Part model, mm, in its own coordinate system. Face numbers are marked on the shaded views. A direction names the side the tool comes from. Coordinates: 2 decimals unless noted, no trailing zeros. Loops run counter-clockwise (first coordinate to the right, second up) from the corner with the lowest first, then second, coordinate; pieces in that order, holes last. Notation, with made-up numbers: (48.25, 19) -> (99.25, 19) arc R34 ccw to (99.25, 53) -> close; hole circle Ø4 at (-21, 12). An arc over 180 degrees is marked (long way). One line per question, with ' | ' between items. Start each with the question number.
1) Cut at A-A (x = 13.5). List the corners of the cut face in (y, z), plus the area to 3 significant figures.
2) Two-plate mould, pull along Y, no slides. Class the marked faces 4, 5 and 6: released by +Y, released by -Y, zero draft, split by the parting line, or undercut.
3) Drop flat-ended pins along their axis: pin 1 (4 mm diameter, centred on y = -13.5, z = 3, fed in from +X); pin 2 (9.5 mm diameter, centred on x = 64.5, z = -1.5, fed in from +Y); pin 3 (13 mm diameter, centred on x = 67.5, z = 3, fed in from -Y). Give the stop position or say it passes through.
4) 3-axis set-ups, long thin cutter, end or side, ignore diameter. For the marked faces 1, 2 and 3: which of +Z, -Z, +X, -X, +Y, -Y reach the whole face in a straight line?
5) Cut at B-B (x = 47). List the corners of the cut face in (y, z).
6) Cut at C-C (x = 74). List the corners of the cut face in (y, z), plus the area to 3 significant figures.
7) Probe L1, parallel to Y at x = 5, z = 0; L2, parallel to Y at x = 60.5, z = 1; L3, parallel to Y at x = 20, z = -3.5. List the from-to ranges inside material, lowest first. Write a range as from..to.
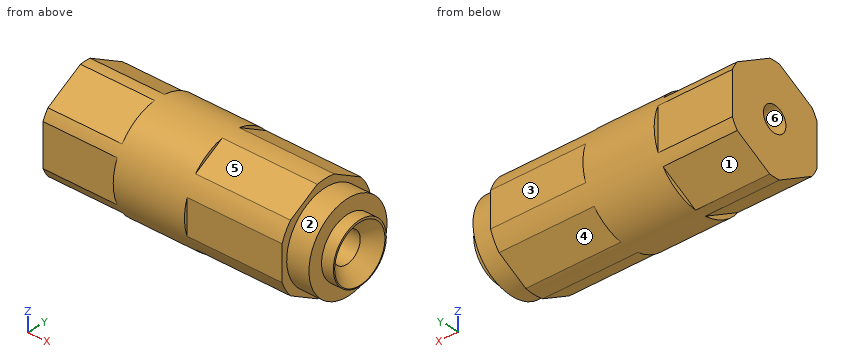
from build123d import *

# Parameters (mm, degrees)
SKETCH5_OUTSIDE_W                 = 57.982
SKETCH5_OUTSIDE_H                 = 57.982
CUT_EXTRUDE3_DEPTH                = 25
M10X1_5_TAPPED_HOLE1_D            = 8.5
M10X1_5_TAPPED_HOLE1_DEPTH        = 24.5
M10X1_5_TAPPED_HOLE1_TIP          = 2.553657631
SKETCH9_OUTSIDE_W                 = 57.982
SKETCH9_OUTSIDE_H                 = 57.982
CUT_EXTRUDE5_DEPTH                = 32
M12X1_75_TAPPED_HOLE1_D           = 10.2
M12X1_75_TAPPED_HOLE1_DEPTH       = 29.25
M12X1_75_TAPPED_HOLE1_CSINK_D     = 19
M12X1_75_TAPPED_HOLE1_CSINK_ANGLE = 90
M12X1_75_TAPPED_HOLE1_TIP         = 3.064389157


with BuildPart() as part:
    # Sketch1 → Revolve1 (revolve)
    with BuildSketch(Plane.XY, mode=Mode.PRIVATE) as revolve1_sk:
        Polygon((0, 0), (0, 17.5), (81, 17.5), (81, 14.75), (88.5, 14.75), (88.5, 10), (92.5, 10), (92.5, 0), (81, 0), align=None)
    revolve(revolve1_sk.sketch.rotate(Axis((0, 0, 0), (-1, 0, 0)), 90), axis=Axis((0, 0, 0), (-1, 0, 0)))

    # Sketch5 outside → Cut-Extrude3 (cut)
    with BuildSketch(Plane.ZY):
        Rectangle(SKETCH5_OUTSIDE_W, SKETCH5_OUTSIDE_H)
        Polygon((9.237604307, 16), (-9.237604307, 16), (-18.475208614, 0), (-9.237604307, -16), (9.237604307, -16), (18.475208614, 0), align=None, mode=Mode.SUBTRACT)
    extrude(amount=-CUT_EXTRUDE3_DEPTH, mode=Mode.SUBTRACT)

    # M10x1.5 Tapped Hole1
    with Locations(Plane.ZY):
        with Locations((0, 0)):
            Hole(M10X1_5_TAPPED_HOLE1_D / 2, depth=M10X1_5_TAPPED_HOLE1_DEPTH)
            with Locations((0, 0, -(M10X1_5_TAPPED_HOLE1_DEPTH + M10X1_5_TAPPED_HOLE1_TIP / 2))):  # 118° drill point
                Cone(0, M10X1_5_TAPPED_HOLE1_D / 2, M10X1_5_TAPPED_HOLE1_TIP, mode=Mode.SUBTRACT)

    # Sketch9 outside → Cut-Extrude5 (cut)
    with BuildSketch(Plane(origin=(81, 0, 0), x_dir=(0, 0, -1), z_dir=(1, 0, 0))):
        Rectangle(SKETCH9_OUTSIDE_W, SKETCH9_OUTSIDE_H)
        Polygon((-9.526279442, -16.5), (9.526279442, -16.5), (19.052558883, 0), (9.526279442, 16.5), (-9.526279442, 16.5), (-19.052558883, 0), align=None, mode=Mode.SUBTRACT)
    extrude(amount=-CUT_EXTRUDE5_DEPTH, mode=Mode.SUBTRACT)

    # M12x1.75 Tapped Hole1
    with Locations(Plane(origin=(92.5, 0, 0), x_dir=(0, 0, -1), z_dir=(1, 0, 0))):
        with Locations((0.231792895, -0.025036362)):
            CounterSinkHole(M12X1_75_TAPPED_HOLE1_D / 2, M12X1_75_TAPPED_HOLE1_CSINK_D / 2, depth=M12X1_75_TAPPED_HOLE1_DEPTH, counter_sink_angle=M12X1_75_TAPPED_HOLE1_CSINK_ANGLE)
            with Locations((0, 0, -(M12X1_75_TAPPED_HOLE1_DEPTH + M12X1_75_TAPPED_HOLE1_TIP / 2))):  # 118° drill point
                Cone(0, M12X1_75_TAPPED_HOLE1_D / 2, M12X1_75_TAPPED_HOLE1_TIP, mode=Mode.SUBTRACT)


solid = part.part
Reported:
1) outline: (-16, -7.09) arc R17.5 ccw to (-14.14, -10.31) -> (-1.86, -17.4) arc R17.5 ccw to (1.86, -17.4) -> (14.14, -10.31) arc R17.5 ccw to (16, -7.09) -> (16, 7.09) arc R17.5 ccw to (14.14, 10.31) -> (1.86, 17.4) arc R17.5 ccw to (-1.86, 17.4) -> (-14.14, 10.31) arc R17.5 ccw to (-16, 7.09) -> close; hole circle Ø8.5 at (0, 0) | area: 820 mm²
2) face 4: released by +Y | face 5: released by -Y | face 6: undercut
3) pin 1: stops at x = 88.5 | pin 2: stops at y = 16.5 | pin 3: stops at y = -16.5
4) face 1: -Z, -X, +Y | face 2: +X | face 3: +Z, -Z, +X, +Y
5) outline: circle Ø35 at (0, 0)
6) outline: (-16.5, -5.83) arc R17.5 ccw to (-13.3, -11.37) -> (-3.2, -17.2) arc R17.5 ccw to (3.2, -17.2) -> (13.3, -11.37) arc R17.5 ccw to (16.5, -5.83) -> (16.5, 5.83) arc R17.5 ccw to (13.3, 11.37) -> (3.2, 17.2) arc R17.5 ccw to (-3.2, 17.2) -> (-13.3, 11.37) arc R17.5 ccw to (-16.5, 5.83) -> close; hole circle Ø10.2 at (-0.03, -0.23) | area: 833 mm²
7) L1: y = -16..-4.25, 4.25..16 | L2: y = -16.5..16.5 | L3: y = -16..-2.41, 2.41..16
